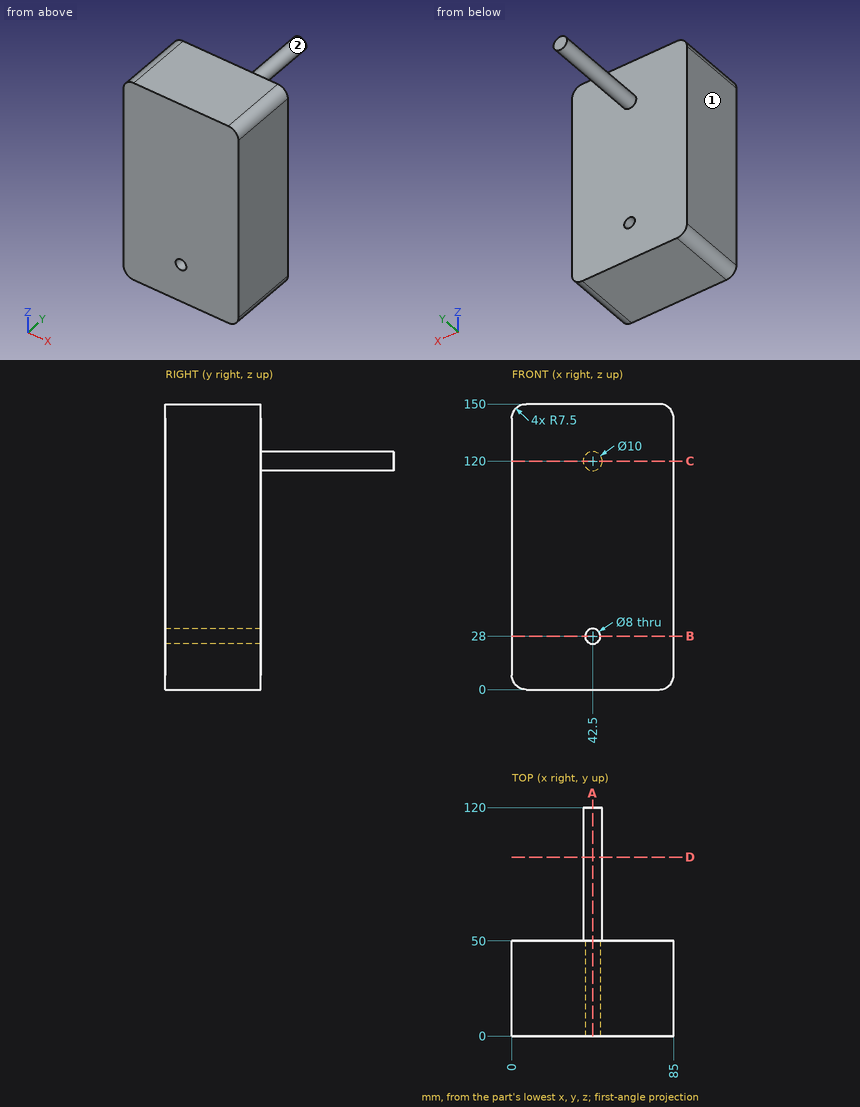
Input: dimensioned drawing with shaded views. Units: mm. Origin: part minimum x, y, z. A direction names the side the tool comes from. Round coordinates to 2 decimals unless told otherwise and drop trailing zeros. Loops run counter-clockwise (first coordinate to the right, second up) from the corner with the lowest first, then second, coordinate; pieces in that order, holes last. Notation, with made-up numbers: (54, 49.5) -> (85, 49.5) arc R20 ccw to (85, 68.5) -> close; hole circle Ø6 at (50.5, 4). An arc over 180 degrees is marked (long way). Answer as a JSON object with one key per item and string values. Group by question number.
1) Ray query, L1, parallel to Z at x = 42.5, y = 23; L2, parallel to X at y = 21, z = 28; L3, parallel to Y at x = 7, z = 65.5. Return the intervals inside material, ascending.
2) Pin query (flat end, axial travel): pin 1 (1 mm diameter, centred on x = 48.5, z = 73, fed in from +Y). Return the tip coordinate at first contact, or that it passes through.
3) Section query D-D on y = 94. Output: boundary loops of the cut face in (x, z), plus the area to 3 significant figures.
4) Section query B-B on z = 28. Output: boundary loops of the cut face in (x, y).
5) Reachability of the marked faces 1 and 2 from +Z, -Z, +X, -X, +Y, -Y: full face, straight path, thin tool, end or side. Return the list, or none.
6) Section query C-C on z = 120. Output: boundary loops of the cut face in (x, y), plus the area to 3 significant figures.
7) Section query A-A on x = 42.5. Output: boundary loops of the cut face in (y, z), plus the area to 3 significant figures.
Reply:
{
 "1": {"L1": "z = 0 to 24, 32 to 150", "L2": "x = 0 to 38.5, 46.5 to 85", "L3": "y = 0 to 50"},
 "2": {"pin 1": "stops at y = 50"},
 "3": {"outline": "circle Ø10 at (42.5, 120)", "area": "78.5 mm2"},
 "4": {"outline": "(0, 0) -> (38.5, 0) -> (38.5, 50) -> (0, 50) -> close; (46.5, 0) -> (85, 0) -> (85, 50) -> (46.5, 50) -> close"},
 "5": {"face 1": "+Z, -Z, -X, +Y, -Y", "face 2": "+Y"},
 "6": {"outline": "(0, 0) -> (85, 0) -> (85, 50) -> (47.5, 50) -> (47.5, 120) -> (37.5, 120) -> (37.5, 50) -> (0, 50) -> close", "area": "4,950 mm2"},
 "7": {"outline": "(0, 0) -> (50, 0) -> (50, 24) -> (0, 24) -> close; (0, 32) -> (50, 32) -> (50, 115) -> (120, 115) -> (120, 125) -> (50, 125) -> (50, 150) -> (0, 150) -> close", "area": "7,800 mm2"}
}
